The model under review builds one solid part; all positions refer to its coordinate system, in mm. A direction names the side the tool comes from. Coordinates: 2 decimals unless noted, no trailing zeros. Loops run counter-clockwise (first coordinate to the right, second up) from the corner with the lowest first, then second, coordinate; pieces in that order, holes last. Notation, with made-up numbers: M 66,18 L 73,18 A23 ccw 73,28 Z; hole C 54.25,16 d10. An arc over 180 degrees is marked long. Write item = value, one per line. Start each with the question number.
Q1. Clearance check with flat-ended pins moving along their axes: pin 1 Ø5 at (x, y) = (53.5, -12) entering from +Z; pin 2 Ø6 at (x, y) = (-71.5, 4) entering from -Z; pin 3 Ø5 at (y, z) = (1.5, 51) entering from -X. State where each tip first meets the part, or that it passes through.
Q2. We need section A-A on y = -10. Give the boundary of the cut face in (x, z), and give its area (3 significant figures).
Q3. We need section C-C on z = -247.5. Give the boundary of the cut face in (x, y) (1 decimal), and give its area (3 significant figures).
Q4. For faces 1 (the face through (-101.6, -5, 0)), 2 (the face through (9.388, 14.724, -79.045)), 3 (the face through (0, 0, -279.4)), 4 (the face through (61.38, -14.84, -7.73)), 5 (the face through (-61.38, -14.84, -7.73)), list the 3-axis set-ups (+Z, -Z, +X, -X, +Y, -Y) from which the entire face can be reached by the end or side of a thin tool; tool diameter is ignored.
Q5. Wall thickness on probe 1 along Z at (x, y) = (23, -5.5); probe 2 along Z at (x, y) = (-44, -7); probe 3 along X at (y, z) = (13, -109): over which ranges is each line inside the solid? List them lowest first.
Q6. We need section B-B on x = 64. Give the boundary of the cut face in (y, z).
Q7. We need section D-D on z = -7.5. Give the boundary of the cut face in (x, y) (1 decimal).
from build123d import *

# Parameters (mm, degrees)
F0_R      = 17.4625
F1_DEPTH  = 279.4
F1_FACE_R = 17.4625
F2_DEPTH  = 127
F3_R      = 12.7
F4_DEPTH  = 101.6
F5_DEPTH  = 101.6


with BuildPart() as f1:
    # F0 (on Top) → F1 (new body)
    with BuildSketch(Plane.XY):
        Circle(F0_R)
    extrude(amount=-F1_DEPTH)

    # F1_face (on face) → F2 (join)
    with BuildSketch(Plane.XY):
        Circle(F1_FACE_R)
    extrude(amount=F2_DEPTH)

    # F3 (on Right) → F4 (join)
    with BuildSketch(Plane.YZ):
        with Locations((-4.7625, 0)):
            Circle(F3_R)
    extrude(amount=F4_DEPTH)

    # F3 (on Right) → F5 (join)
    with BuildSketch(Plane.YZ):
        with Locations((-4.7625, 0)):
            Circle(F3_R)
    extrude(amount=-F5_DEPTH)


solid = f1.part
Returned:
q1.pin_1 = 11.78
q1.pin_2 = -11.32
q1.pin_3 = -17.46
q2.outline = M -101.6,-11.57 L -14.32,-11.57 L -14.32,-279.4 L 14.32,-279.4 L 14.32,-11.57 L 101.6,-11.57 L 101.6,11.57 L 14.32,11.57 L 14.32,127 L -14.32,127 L -14.32,11.57 L -101.6,11.57 Z
q2.area = 15,700 mm^2
q3.outline = C 0,0 d34.9
q3.area = 958 mm^2
q4.face_1 = +Z, -Z, -X, +Y, -Y
q4.face_2 = none
q4.face_3 = -Z, +X, -X, +Y, -Y
q4.face_4 = +X
q4.face_5 = -X
q5.probe_1 = -12.68 to 12.68
q5.probe_2 = -12.5 to 12.5
q5.probe_3 = -11.66 to 11.66
q6.outline = C -4.76,0 d25.4
q7.outline = M -101.6,-15 L -8.9,-15 A17.5 ccw 8.9,-15 L 101.6,-15 L 101.6,5.5 L 16.6,5.5 A17.5 ccw -16.6,5.5 L -101.6,5.5 Z
